Part model, mm, in its own coordinate system. Give positions to 0.01 mm unless a question says otherwise; leave off trailing zeros. Order: outer loops, then holes, each group sorted by start corner. A loop starts at its lowest first (then second) coordinate and runs counter-clockwise, first axis right, second up.
1. Drop a flat-ended pin along its axis: pin 1 Ø1.5 at (x, y) = (23, 5) entering from -Z. Give the stop position or say it passes through.
2. Slice it at B-B on x = -59. List the corners of the cut face in (y, z).
3. Probe line 1 (X direction, y = 3.5, z = 0); line 2 (X direction, y = 6, z = 25); line 3 (Z direction, x = 28, y = 6). List the from-to ranges inside material, lowest first.
4. Slice it at D-D on z = 51. List the corners of the cut face in (x, y).
5. Slice it at A-A on y = 3.75. Give the number of separate pieces and of enclosed holes in the cut face, and give its area (3 significant figures).
6. Slice it at C-C on x = -4. List the corners of the cut face in (y, z), and give its area (3 significant figures).
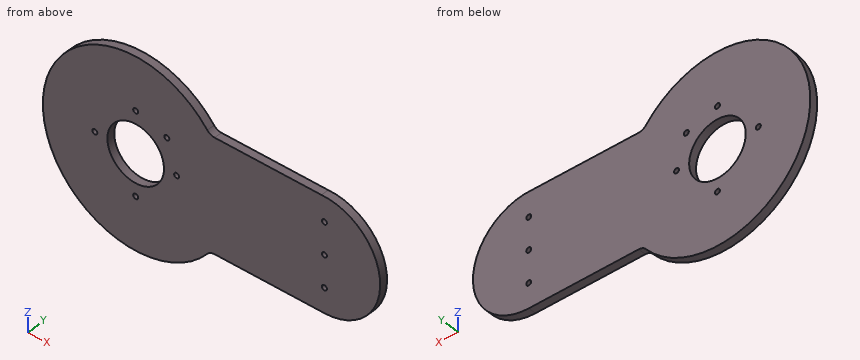
from build123d import *

# Parameters (mm, degrees)
SKETCH1_R                   = 2.0193
BOSS_EXTRUDE1_DEPTH         = 6.35
SKETCH16_R                  = 22.86
SKETCH16_R_2                = 2.0193
CUT_EXTRUDE1_DEPTH          = 6.35
FILLET1_R                   = 7.62
F_21_0_159_DIAMETER_HOLE1_D = 4.0386


with BuildPart() as part:
    # Sketch1 → Boss-Extrude1 (new body)
    with BuildSketch(Plane(origin=(0, 0, 0), x_dir=(1, 0, 0), z_dir=(0, 1, 0))):
        with BuildLine():
            Line((75, -45), (-14.998600006, -45))
            ThreePointArc((-14.998600006, -45), (-150.00112, 0), (-14.998600006, 45))
            Line((-14.998600006, 45), (77.4, 45.063954554))
            ThreePointArc((77.4, 45.063954554), (122.447963078, -1.200425985), (75, -45))
        make_face()
        with Locations(Location((77.4, 0, 0), (0, 0, 270))):
            Circle(SKETCH1_R, mode=Mode.SUBTRACT)
    extrude(amount=BOSS_EXTRUDE1_DEPTH)

    # Sketch16 → Cut-Extrude1 (cut)
    with BuildSketch(Plane(origin=(0.964771866, 6.35, 105.934324836), x_dir=(-1, 0, 0), z_dir=(0, 1, 0))):
        with Locations(Location((75.964771866, -105.934324836, 0), (0, 0, 90))):
            Circle(SKETCH16_R)
        with Locations(Location((50.800979112, -80.770532082, 0), (0, 0, 90))):
            Circle(SKETCH16_R_2)
        with Locations(Location((42.944771866, -105.934324836, 0), (0, 0, 90))):
            Circle(SKETCH16_R_2)
        with Locations(Location((75.964771866, -72.914324836, 0), (0, 0, 90))):
            Circle(SKETCH16_R_2)
        with Locations(Location((108.984771866, -105.934324836, 0), (0, 0, 90))):
            Circle(SKETCH16_R_2)
        with Locations(Location((75.964771866, -138.954324836, 0), (0, 0, 90))):
            Circle(SKETCH16_R_2)
    extrude(amount=-CUT_EXTRUDE1_DEPTH, mode=Mode.SUBTRACT)

    # Fillet1
    fillet1_edges = [part.edges().sort_by_distance(p)[0] for p in [
        (-14.998600006, 3.175, -45),
        (-14.998600006, 3.175, 45),
    ]]
    fillet(fillet1_edges, radius=FILLET1_R)

    # #21 (0.159) Diameter Hole1 (through all)
    with Locations(Plane(origin=(0, 6.35, 0), x_dir=(1, 0, 0), z_dir=(0, 1, 0))):
        with Locations((77.4, 25.4), (77.4, -25.4)):
            Hole(F_21_0_159_DIAMETER_HOLE1_D / 2)


solid = part.part
Data:
1. pin 1: stops at z = -45.03
2. outline: (0, -73.27) - (6.35, -73.27) - (6.35, -16.33) - (0, -16.33) - close; (0, 16.33) - (6.35, 16.33) - (6.35, 73.27) - (0, 73.27) - close
3. line 1: x = -150 to -110.04, -106 to -97.86, -52.14 to -44, -39.96 to 75.38, 79.42 to 122.46
3. line 2: x = -145.71 to -51.85, -47.82 to 75.42, 79.38 to 114.89
3. line 3: z = -45.03 to 45
4. outline: (-129.99, 0) - (-20.01, 0) - (-20.01, 6.35) - (-129.99, 6.35) - close
5. separate pieces: 1
5. enclosed holes: 9
5. area: 26,500 mm2
6. outline: (0, -45.01) - (6.35, -45.01) - (6.35, 45) - (0, 45) - close
6. area: 572 mm2
